Geometry check sheet. Reference: the model listing, model coordinates, mm. Coordinates: 2 decimals unless noted, no trailing zeros. Write each loop counter-clockwise with the first axis right and the second up, starting at its lowest first coordinate (ties: lowest second). Pieces come first, ordered by that corner, then holes. Notation, with made-up numbers: (63.5, 55) -> (83.5, 55) arc R24 cw to (83.5, 67) -> close; hole circle Ø6 at (47.25, -9.75). An arc over 180 degrees is marked (long way). One line per question, with ' | ' between items.
Autodesk Inventor part; units mm, degrees
ref_plane "YZ Plane" through (0, 0, 0) normal (1, 0, 0) x (0, 1, 0)
ref_plane "XZ Plane" through (0, 0, 0) normal (0, 1, 0) x (-1, 0, 0)
ref_plane "XY Plane" through (0, 0, 0) normal (0, 0, 1) x (1, 0, 0)
sketch "Sketch1" plane through (0, 0, 0) normal (0, 0, 1) x (1, 0, 0)
  line L0 (-272, -28) -> (272, -28)
  line L1 (300, 0) -> (300, 28)
  line L2 (300, 28) -> (-272, 28) construction
  line L3 (-300, 0) -> (-300, 0)
  line L4 (-300, -28) -> (300, 28) construction
  line L5 (300, -28) -> (-300, 28) construction
  arc A0 (-272, 28) -> (-300, 0) centre (-272, 0) ccw
  arc A1 (-300, 0) -> (-272, -28) centre (-272, 0) ccw
  circle A2 centre (-152, 0) radius 7
  circle A3 centre (-162.6066, 10.6066) radius 1.5
  line L6 (-152, 0) -> (-162.6066, 10.6066) construction
  line L7 (-152, 0) -> (-272, 0) construction
  circle A4 centre (-162.6066, -10.6066) radius 1.5
  circle A5 centre (-141.3934, -10.6066) radius 1.5
  circle A6 centre (-141.3934, 10.6066) radius 1.5
  arc A7 (272, -28) -> (300, 0) centre (272, 0) ccw
  circle A8 centre (272, 0) radius 7
  line L8 (300, 28) -> (300, 84)
  line L9 (300, 84) -> (244, 84)
  line L10 (244, 84) -> (244, 28)
  line L11 (244, 28) -> (-272, 28)
  circle A9 centre (272, 56) radius 7
  circle A10 centre (-272, 0) radius 7
  circle A11 centre (-280, 8) radius 2
  circle A12 centre (-280, -8) radius 2
  circle A13 centre (-264, -8) radius 2
  circle A14 centre (-264, 8) radius 2
  point P0 (0, 0)
  point P1 (-300, 0)
  dimension "d0" = 600
  dimension "d1" = 56
  dimension "d3" = 28
  dimension "d4" = 14
  dimension "d5" = 120
  dimension "d6" = 3
  dimension "d7" = 45
  dimension "d8" = 15
  dimension "d11" = 360
  dimension "d13" = 28
  dimension "d16" = 14
  dimension "d17" = 56
  dimension "d18" = 56
  dimension "d19" = 14
  dimension "d20" = 56
  dimension "d21" = 14
  dimension "d22" = 4
  dimension "d23" = 8
  dimension "d24" = 8
  dimension "d27" = 360
extrude "Extrusion1" add sketch "Sketch1" along normal blind 3.175
sketch "Sketch2" plane through (0, 0, 3.175) normal (0, 0, 1) x (1, 0, 0)
  line L0 (244, 28) -> (-272, 28) construction
  circle A0 centre (-272, 24) radius 2
  circle A1 centre (-248, 24) radius 2
  circle A2 centre (-224, 24) radius 2
  circle A3 centre (-200, 24) radius 2
  circle A4 centre (-176, 24) radius 2
  circle A5 centre (-152, 24) radius 2
  circle A6 centre (-128, 24) radius 2
  circle A7 centre (-104, 24) radius 2
  circle A8 centre (-80, 24) radius 2
  circle A9 centre (-56, 24) radius 2
  circle A10 centre (-32, 24) radius 2
  circle A11 centre (-8, 24) radius 2
  line L1 (0, 28) -> (0, -28) construction
  line L2 (-272, -28) -> (272, -28) construction
  circle A12 centre (272, 24) radius 2
  circle A13 centre (248, 24) radius 2
  circle A14 centre (224, 24) radius 2
  circle A15 centre (200, 24) radius 2
  circle A16 centre (176, 24) radius 2
  circle A17 centre (152, 24) radius 2
  circle A18 centre (128, 24) radius 2
  circle A19 centre (104, 24) radius 2
  circle A20 centre (80, 24) radius 2
  circle A21 centre (56, 24) radius 2
  circle A22 centre (32, 24) radius 2
  circle A23 centre (8, 24) radius 2
  arc A24 (-272, 28) -> (-272, -28) centre (-272, 0) ccw construction
  arc A25 (272, -28) -> (300, 0) centre (272, 0) ccw construction
  line L3 (-300, 0) -> (300, 0) construction
  line L4 (244, -28) -> (-272, -28) construction
  circle A26 centre (-272, -24) radius 2
  circle A27 centre (-248, -24) radius 2
  circle A28 centre (-224, -24) radius 2
  circle A29 centre (-200, -24) radius 2
  circle A30 centre (-176, -24) radius 2
  circle A31 centre (-152, -24) radius 2
  circle A32 centre (-128, -24) radius 2
  circle A33 centre (-104, -24) radius 2
  circle A34 centre (-80, -24) radius 2
  circle A35 centre (-56, -24) radius 2
  circle A36 centre (-32, -24) radius 2
  circle A37 centre (-8, -24) radius 2
  circle A38 centre (80, -24) radius 2
  circle A39 centre (56, -24) radius 2
  circle A40 centre (32, -24) radius 2
  circle A41 centre (8, -24) radius 2
  circle A42 centre (104, -24) radius 2
  circle A43 centre (128, -24) radius 2
  circle A44 centre (152, -24) radius 2
  circle A45 centre (176, -24) radius 2
  circle A46 centre (200, -24) radius 2
  circle A47 centre (224, -24) radius 2
  circle A48 centre (248, -24) radius 2
  circle A49 centre (272, -24) radius 2
  circle A50 centre (248, 80) radius 2
  line L5 (244, 84) -> (244, 28) construction
  line L6 (300, 84) -> (244, 84) construction
  circle A51 centre (296, 80) radius 2
  line L7 (300, 0) -> (300, 84) construction
  circle A52 centre (248, 52) radius 2
  circle A53 centre (296, 52) radius 2
  point P0 (0, 0)
  point P1 (272, 28)
  dimension "d29" = 4
  dimension "d30" = 4
  dimension "d33" = 24
  dimension "d38" = 4
  dimension "d39" = 4
  dimension "d40" = 4
  dimension "d41" = 4
  dimension "d42" = 4
  dimension "d43" = 4
  dimension "d44" = 4
  dimension "d45" = 28
  dimension "d46" = 4
extrude "Extrusion2" cut sketch "Sketch2" against normal through all
equation "\"d3\" = 0.5 * d1"
equation "\"d13\" = d3"
properties part number "FirstStageArmBar1"
(1) Cross-section at B-B (x = -233.5). Record the cut outline in (y, z) (3 decimals), plus the area to 3 significant figures.
Answers below:
outline: (-28, 0) -> (28, 0) -> (28, 3.175) -> (-28, 3.175) -> close | area: 178 mm²
(2) Cross-section at C-C (z = 1.1). Count the separate pieces of the cut face and the enclosed holes in it, plus the area to 3 significant figures.
Answers below:
separate pieces: 1 | enclosed holes: 64 | area: 34,900 mm²
(3) Material ranges on line 1 (X direction, y = 1, z = 1.95); line 2 (Y direction, x = -152, z = 1.3); line 3 (Y direction, x = 80.5, z = 0.95), recorded low to high.
Answers below:
line 1: x = -299.98 to -278.93, -265.07 to -158.93, -145.07 to 265.07, 278.93 to 300 | line 2: y = -28 to -26, -22 to -7, 7 to 22, 26 to 28 | line 3: y = -28 to -25.94, -22.06 to 22.06, 25.94 to 28
(4) Cross-section at A-A (y = 71). Record the cut outline in (x, z) (3 decimals).
Answers below:
outline: (244, 0) -> (300, 0) -> (300, 3.175) -> (244, 3.175) -> close
(5) Draft check along Y on faces 1 (the face through (292.015, -19.58, 1.565)), 2 (the face through (-299.993, -0.616, 1.565)), 3 (the face through (-265.323, -2.103, 1.565)). Enter one of: pulls with the +Y half, pulls with the -Y half, needs draft (parallel to the pull), parting line crosses it, or undercut.
Answers below:
face 1: pulls with the -Y half | face 2: parting line crosses it | face 3: undercut
(6) Depth check by flat-ended pin: P1, Ø3, axis at x = -176, y = -24, coming from the +Z side. Enter the tip coordinate at first touch or a pass-through.
Answers below:
P1: passes through
